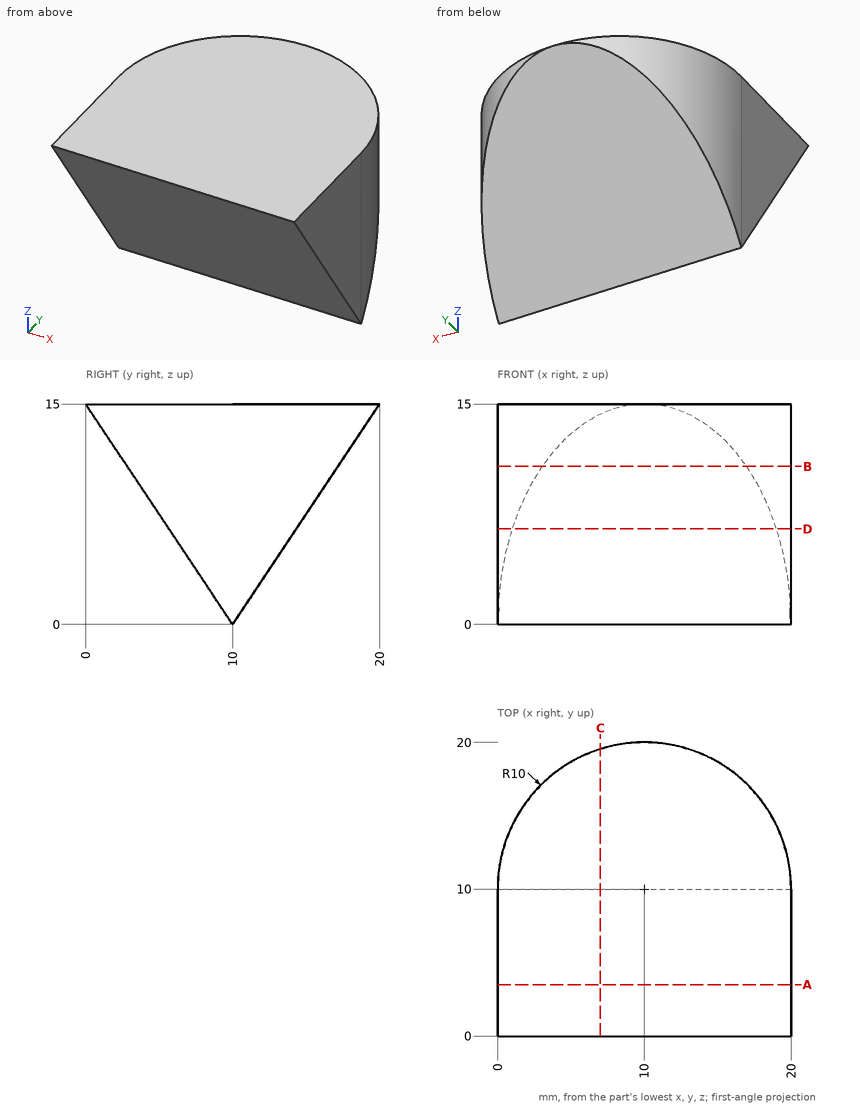
Part print with two shaded views. Sizes in mm from the minimum x, y, z corner. Give positions to 0.01 mm unless a question says otherwise; leave off trailing zeros. Order: outer loops, then holes, each group sorted by start corner. A loop starts at its lowest first (then second) coordinate and runs counter-clockwise, first axis right, second up. Notation, with made-up numbers: M 26.25,-15.75 L 51.25,-15.75 A19 ccw 51.25,-6.75 Z; hole C -23,-13 d1. An arc over 180 degrees is marked long. Put each result on its own line as item: value.
Item 1: Cut at A-A on y = 3.5. Write the cut outline in (x, z).
Results are:
outline: M 0,9.75 L 20,9.75 L 20,15 L 0,15 Z
Item 2: Cut at D-D on z = 6.5. Write the cut outline in (x, y), then the cut area to 3 significant figures.
Results are:
outline: M 0,5.67 L 20,5.67 L 20,10 A10 ccw 19.01,14.33 L 0.99,14.33 A10 ccw 0,10 Z
area: 171 mm2
Item 3: Cut at C-C on x = 7. Write the cut outline in (y, z).
Results are:
outline: M 0,15 L 10,0 L 19.54,14.31 L 19.54,15 Z
Item 4: Drop flat-ended pins along their axis: pin 1 Ø1.5 at (x, y) = (17, 15) entering from -Z (3 decimals); pin 2 Ø1.5 at (x, y) = (13, 12.5) entering from -Z (3 decimals). Give the stop position or say it passes through.
Results are:
pin 1: z = 6.375
pin 2: z = 2.625
Item 5: Wall check: probe 1 along Z at (x, y) = (4.5, 1.5); probe 2 along Y at (x, z) = (7, 7.5); probe 3 along Y at (x, z) = (17.75, 8.5). Give the ranges that are in metal, low to high.
Results are:
probe 1: 12.75 to 15
probe 2: 5 to 15
probe 3: 4.33 to 15.67
Item 6: Cut at B-B on z = 10.75. Write the cut outline in (x, y), then the cut area to 3 significant figures.
Results are:
outline: M 0,2.83 L 20,2.83 L 20,10 A10 ccw 16.97,17.17 L 3.03,17.17 A10 ccw 0,10 Z
area: 273 mm2
